The figure shows three views and two pictorial views of one solid part (mm, origin at its lowest corner). Answer the questions. A direction names the side the tool comes from. Round coordinates to 2 decimals unless told otherwise and drop trailing zeros. Loops run counter-clockwise (first coordinate to the right, second up) from the corner with the lowest first, then second, coordinate; pieces in that order, holes last. Notation, with made-up numbers: (44.25, 25.5) -> (96.25, 25.5) arc R21 ccw to (96.25, 47.5) -> close; hole circle Ø1 at (-2, 5.25). An arc over 180 degrees is marked (long way). Use a Markdown table: item, result. Add a question column.
Q1. Given pin 1 Ø1 at (x, y) = (16, 30.5) entering from +Z; pin 2 Ø2 at (y, z) = (31.5, 4.5) entering from +X; pin 3 Ø2 at (y, z) = (31.5, 4) entering from -X, each flat-ended and moving along its own axis, determine where each tip first touches the part or whether it passes through.
Q2. Consider line 1 (Z direction, x = 12, y = 27.5); line 2 (Y direction, x = 42, z = 33.5); line 3 (Y direction, x = 13, z = 21) (1 decimal). Determine where each line is inside the solid, lowest interval first.
Q3. Section A-A on x = 16 is taken. Give the vertices of the cut face in (y, z) (1 decimal).
Q4. Section B-B on z = 15.5 is taken. Give the vertices of the cut face in (x, y) (1 decimal).
Q5. Section C-C on y = 26 is taken. Give the vertices of the cut face in (x, z) (1 decimal), then the cut area to 3 significant figures.
Q6. Which of the six approach directions +Z, -Z, +X, -X, +Y, -Y give full straight-line access (tool end or side, diameter ignored) to the marked faces 1 and 2?
Q7. Section D-D on x = 30 is taken. Give the vertices of the cut face in (y, z) (1 decimal).
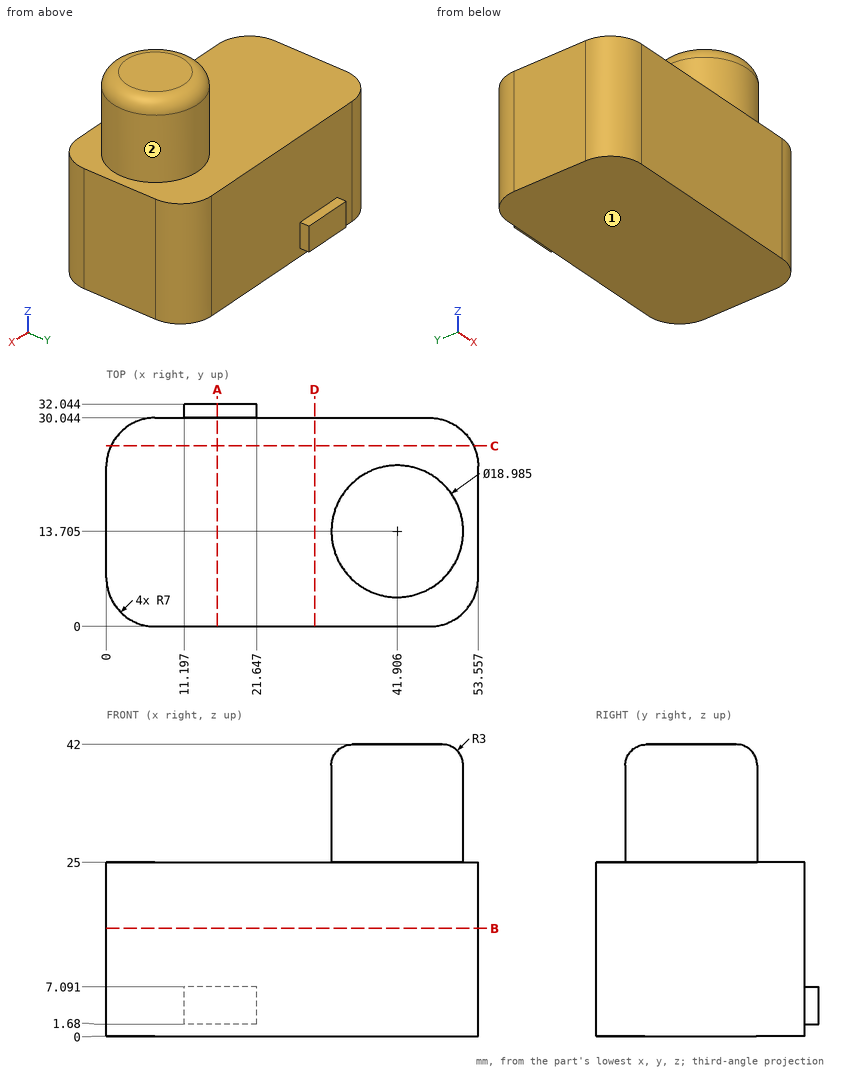
Checked values:
| question | item | result |
|---|---|---|
| 1 | pin 1 | stops at z = 25 |
| 1 | pin 2 | stops at x = 21.65 |
| 1 | pin 3 | stops at x = 11.2 |
| 2 | line 1 | z = 0 to 25 |
| 2 | line 2 | y = 4.21 to 23.2 |
| 2 | line 3 | y = 0 to 30 |
| 3 | outline | (0, 0) -> (30, 0) -> (30, 1.7) -> (32, 1.7) -> (32, 7.1) -> (30, 7.1) -> (30, 25) -> (0, 25) -> close |
| 4 | outline | (0, 7) arc R7 ccw to (7, 0) -> (46.6, 0) arc R7 ccw to (53.6, 7) -> (53.6, 23) arc R7 ccw to (46.6, 30) -> (7, 30) arc R7 ccw to (0, 23) -> close |
| 5 | outline | (0.7, 0) -> (52.9, 0) -> (52.9, 25) -> (0.7, 25) -> close |
| 5 | area | 1,310 mm2 |
| 6 | face 1 | -Z, +X, -X, +Y, -Y |
| 6 | face 2 | +Z |
| 7 | outline | (0, 0) -> (30, 0) -> (30, 25) -> (0, 25) -> close |
